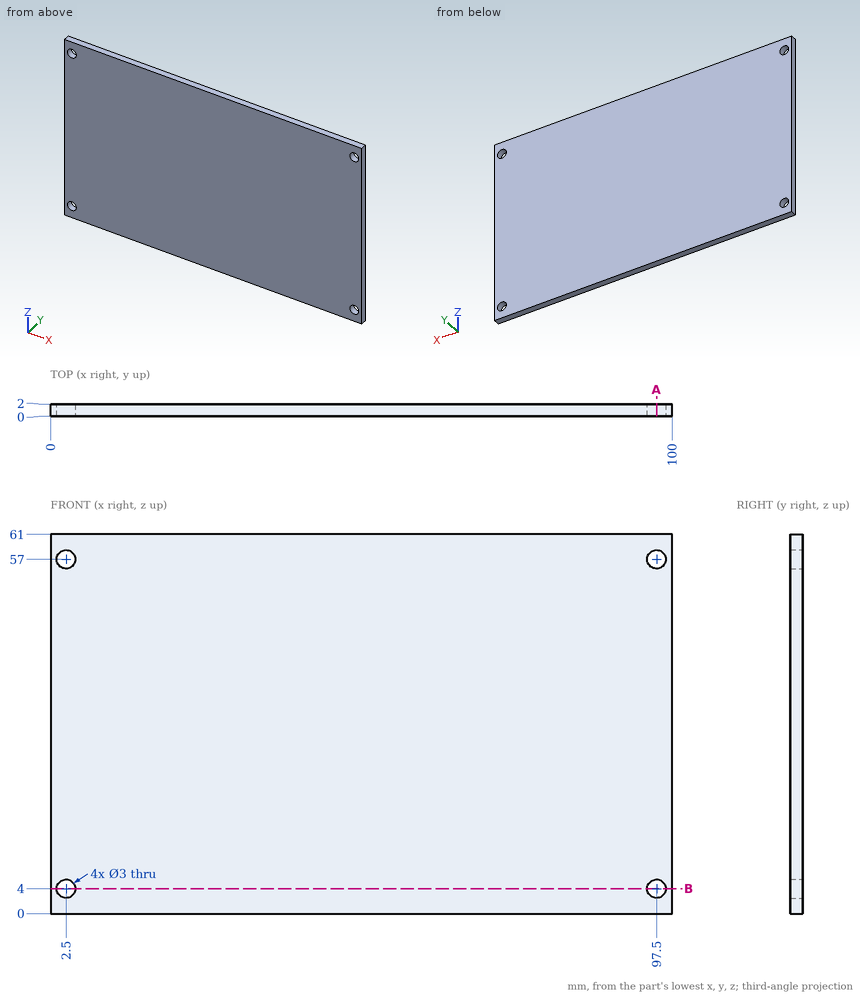
Verification items for this drawing (mm, ordinates from the low corner). Give positions to 0.01 mm unless a question says otherwise; leave off trailing zeros. Loops run counter-clockwise (first coordinate to the right, second up) from the corner with the lowest first, then second, coordinate; pieces in that order, holes last. Notation, with made-up numbers: M 52.5,-11.5 L 60.5,-11.5 A30 ccw 60.5,15.5 Z; hole C 16,29.25 d11. An arc over 180 degrees is marked long. Answer as a JSON object with one key per item and string values. Group by question number.
Item 1: Gauge pin test, flat end, axial feed: pin 1 (1.8 mm diameter, centred on x = 97.5, z = 4, fed in from +Y). Record the tip position at first contact, or that the pin passes through.
Item 2: Material ranges on L1, parallel to X at y = 0.6, z = 4; L2, parallel to Z at x = 2.5, y = 1.6, recorded low to high.
Item 3: Sectioned sample at A-A on x = 97.5. Record the boundary of the cut face in (y, z), plus the area to 3 significant figures.
Item 4: Sectioned sample at B-B on z = 4. Record the boundary of the cut face in (x, y), plus the area to 3 significant figures.
Findings below:
{
 "1": {"pin 1": "through"},
 "2": {"L1": "0 to 1, 4 to 96, 99 to 100", "L2": "0 to 2.5, 5.5 to 55.5, 58.5 to 61"},
 "3": {"outline": "M 0,0 L 2,0 L 2,2.5 L 0,2.5 Z; M 0,5.5 L 2,5.5 L 2,55.5 L 0,55.5 Z; M 0,58.5 L 2,58.5 L 2,61 L 0,61 Z", "area": "110 mm2"},
 "4": {"outline": "M 0,0 L 1,0 L 1,2 L 0,2 Z; M 4,0 L 96,0 L 96,2 L 4,2 Z; M 99,0 L 100,0 L 100,2 L 99,2 Z", "area": "188 mm2"}
}
